Check sheet for the modelled part. Datum: model origin and axes. Units: mm. Give positions to 0.01 mm unless a question says otherwise; leave off trailing zeros. Write each loop counter-clockwise with the first axis right and the second up, starting at its lowest first coordinate (ties: lowest second). Pieces come first, ordered by that corner, then holes. Notation, with made-up numbers: M 60.5,-35.5 L 113.5,-35.5 A27 ccw 113.5,-2.5 Z; hole C 36,33 d5. An arc over 180 degrees is marked long. Write each question's results on one line, items separated by ' | '. Start each with the question number.
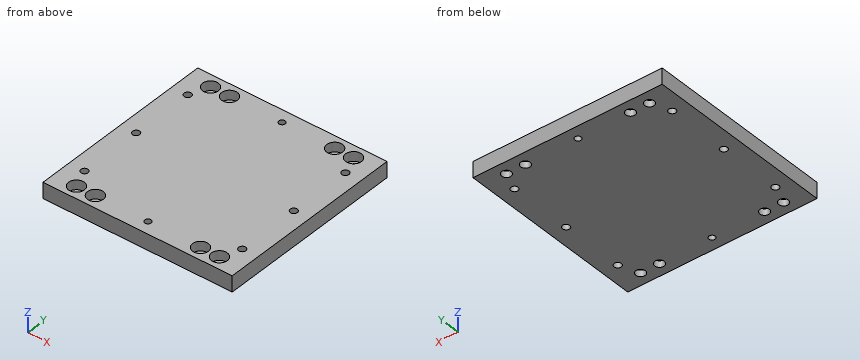
from build123d import *

# Parameters (mm, degrees)
SKETCH_1_W                    = 180
SKETCH_1_H                    = 180
EXTRUDE_1_DEPTH               = 15
HOLE_WIZARD_4_8_1_D           = 9
HOLE_WIZARD_4_8_1_CBORE_D     = 15
HOLE_WIZARD_4_8_1_CBORE_DEPTH = 9
HOLE_WIZARD_6_0_6_1_D         = 6
HOLE_WIZARD_M8_1_D            = 6.8
HOLE_WIZARD_M8_1_DEPTH        = 22.25
HOLE_WIZARD_M8_1_TIP          = 2.042926105


with BuildPart() as part:
    # 草图1 → 凸台-拉伸1 (new body)
    with BuildSketch(Plane.XY):
        Rectangle(SKETCH_1_W, SKETCH_1_H)
    extrude(amount=EXTRUDE_1_DEPTH)

    # 打孔尺寸根据内六角花形圆柱头螺钉-4.8级的类型1 (through all)
    with Locations(Plane(origin=(-68, -78, 15), x_dir=(1, 0, 0), z_dir=(0, 0, 1))):
        with Locations((0, 0), (18, 0), (118, 0), (136, 0), (136, 156), (118, 156), (18, 156), (0, 156)):
            CounterBoreHole(HOLE_WIZARD_4_8_1_D / 2, HOLE_WIZARD_4_8_1_CBORE_D / 2, HOLE_WIZARD_4_8_1_CBORE_DEPTH)

    # Ø6.0 (6) 直径孔1 (through all)
    with Locations(Plane(origin=(0, 78, 15), x_dir=(1, 0, 0), z_dir=(0, 0, 1))):
        with Locations((0, 0), (0, -156)):
            Hole(HOLE_WIZARD_6_0_6_1_D / 2)

    # M8 螺纹孔1
    with Locations(Plane(origin=(-75, 60, 15), x_dir=(1, 0, 0), z_dir=(0, 0, 1))):
        with Locations((0, 0), (0, -60), (0, -120), (150, -120), (150, -60), (150, 0)):
            Hole(HOLE_WIZARD_M8_1_D / 2, depth=HOLE_WIZARD_M8_1_DEPTH)
            with Locations((0, 0, -(HOLE_WIZARD_M8_1_DEPTH + HOLE_WIZARD_M8_1_TIP / 2))):  # 118° drill point
                Cone(0, HOLE_WIZARD_M8_1_D / 2, HOLE_WIZARD_M8_1_TIP, mode=Mode.SUBTRACT)


solid = part.part
Q1. Section check B-B on y = 60. Record the boundary of the cut face in (x, z).
Q2. Section check C-C on z = 8.5. State how many separate pieces and enclosed holes the cut face has, plus the area to 3 significant figures.
Q3. Section check A-A on x = -68. Record the boundary of the cut face in (y, z), plus the area to 3 significant figures.
Q4. Scan lines: L1, parallel to Y at x = 50, z = 4.6; L2, parallel to Y at x = 50, z = 8; L3, parallel to X at y = 82, z = 3. Record each from-to range of solid material in increasing order.
Q5. Section check D-D on x = 0. Record the boundary of the cut face in (y, z).
Q6. Depth check by flat-ended pin: pin 1 Ø13.5 at (x, y) = (68, -78) entering from +Z; pin 2 Ø3.5 at (x, y) = (0, -78) entering from +Z. Enter the tip coordinate at first touch or a pass-through.
Check result:
1) outline: M -90,0 L -78.4,0 L -78.4,15 L -90,15 Z; M -71.6,0 L 71.6,0 L 71.6,15 L -71.6,15 Z; M 78.4,0 L 90,0 L 90,15 L 78.4,15 Z
2) separate pieces: 1 | enclosed holes: 16 | area: 30,700 mm^2
3) outline: M -90,0 L -82.5,0 L -82.5,6 L -85.5,6 L -85.5,15 L -90,15 Z; M -73.5,0 L 73.5,0 L 73.5,6 L 70.5,6 L 70.5,15 L -70.5,15 L -70.5,6 L -73.5,6 Z; M 82.5,0 L 90,0 L 90,15 L 85.5,15 L 85.5,6 L 82.5,6 Z | area: 2,320 mm^2
4) L1: -90 to -82.5, -73.5 to 73.5, 82.5 to 90 | L2: -90 to -85.5, -70.5 to 70.5, 85.5 to 90 | L3: -90 to -70.06, -65.94 to -52.06, -47.94 to 47.94, 52.06 to 65.94, 70.06 to 90
5) outline: M -90,0 L -81,0 L -81,15 L -90,15 Z; M -75,0 L 75,0 L 75,15 L -75,15 Z; M 81,0 L 90,0 L 90,15 L 81,15 Z
6) pin 1: z = 6 | pin 2: through
